```python
from build123d import *

# Parameters (mm, degrees)
ESQUISSE1_W                  = 53
ESQUISSE1_H                  = 38
BASE_DEPTH                   = 4
ESQUISSE2_W                  = 29
ESQUISSE2_H                  = 29
SCREEN_DEPTH                 = 4
ESQUISSE5_R                  = 2.25
INSERTS_M3_DEPTH             = 3
ESQUISSE6_W                  = 53
ESQUISSE6_H                  = 38
ESQUISSE6_W_2                = 50
ESQUISSE6_H_2                = 35
WALLS_DEPTH                  = 25
CHANFREIN_EXT_SIZE           = 1.2
CONG_1_R                     = 1.2
ESQUISSE7_R                  = 1.5
PASSAGE_VIS_HORIZONTAL_DEPTH = 62.603571325
ESQUISSE9_R                  = 1.5
PASSAGE_VIS_VERTICAL_DEPTH   = 53.642663306


with BuildPart() as part:
    # Esquisse1 → BASE (new body)
    with BuildSketch(Plane.XY):
        Rectangle(ESQUISSE1_W, ESQUISSE1_H)
    extrude(amount=BASE_DEPTH)

    # Esquisse2 → Screen (cut)
    with BuildSketch(Plane.XY.offset(4)):
        with Locations((-2.5, 0)):
            Rectangle(ESQUISSE2_W, ESQUISSE2_H)
    extrude(amount=-SCREEN_DEPTH, mode=Mode.SUBTRACT)

    # Esquisse5 → Inserts_M3 (cut)
    with BuildSketch(Plane(origin=(0, 0, 0), x_dir=(-1, 0, 0), z_dir=(0, 0, -1))):
        with Locations((-21, 13.5)):
            Circle(ESQUISSE5_R)
        with Locations(Location((-21, -13.5, 0), (0, 0, 180))):
            Circle(ESQUISSE5_R)
        with Locations((21, -13.5)):
            Circle(ESQUISSE5_R)
        with Locations(Location((21, 13.5, 0), (0, 0, 180))):
            Circle(ESQUISSE5_R)
    extrude(amount=-INSERTS_M3_DEPTH, mode=Mode.SUBTRACT)

    # Esquisse6 → Walls (add)
    with BuildSketch(Plane(origin=(0, 0, 0), x_dir=(-1, 0, 0), z_dir=(0, 0, -1))):
        Rectangle(ESQUISSE6_W, ESQUISSE6_H)
        Rectangle(ESQUISSE6_W_2, ESQUISSE6_H_2, mode=Mode.SUBTRACT)
    extrude(amount=WALLS_DEPTH)

    # Chanfrein_EXT
    chanfrein_ext_edges = [part.edges().sort_by_distance(p)[0] for p in [
        (26.5, 0, 4),
        (0, 19, 4),
        (-17, 0, 4),
        (-2.5, -14.5, 4),
        (12, 0, 4),
        (-2.5, 14.5, 4),
        (-26.5, 0, 4),
        (-26.5, 19, -10.5),
        (26.5, 19, -10.5),
        (26.5, -19, -10.5),
        (-26.5, -19, -10.5),
        (0, -19, 4),
    ]]
    chamfer(chanfrein_ext_edges, length=CHANFREIN_EXT_SIZE)

    # Congé1
    cong_1_edges = [part.edges().sort_by_distance(p)[0] for p in [
        (0, 17.5, 0),
        (25, 0, 0),
        (0, -17.5, 0),
        (-25, 0, 0),
        (25, 17.5, -12.5),
        (25, -17.5, -12.5),
        (-25, -17.5, -12.5),
        (-25, 17.5, -12.5),
    ]]
    fillet(cong_1_edges, radius=CONG_1_R)

    # Esquisse7 → Passage_Vis_Horizontal (cut, through all)
    with BuildSketch(Plane(origin=(26.5, 0, 0), x_dir=(0, 0, -1), z_dir=(1, 0, 0))):
        with Locations(Location((21, 0, 0), (0, 0, 90))):
            Circle(ESQUISSE7_R)
    extrude(amount=-PASSAGE_VIS_HORIZONTAL_DEPTH, mode=Mode.SUBTRACT)

    # Esquisse9 → Passage_Vis_Vertical (cut, through all)
    with BuildSketch(Plane(origin=(0, 19, 0), x_dir=(1, 0, 0), z_dir=(0, 1, 0))):
        with Locations(Location((-18.5, 21, 0), (0, 0, 180))):
            Circle(ESQUISSE9_R)
        with Locations(Location((18.5, 21, 0), (0, 0, 180))):
            Circle(ESQUISSE9_R)
    extrude(amount=-PASSAGE_VIS_VERTICAL_DEPTH, mode=Mode.SUBTRACT)


solid = part.part
```
Can you work these out from the model? Positions are in its coordinate system, mm. A direction names the side the tool comes from. Round coordinates to 2 decimals unless told otherwise and drop trailing zeros. Loops run counter-clockwise (first coordinate to the right, second up) from the corner with the lowest first, then second, coordinate; pieces in that order, holes last.
Item 1: If we mould it in two halves opening along Y, with no side actions, what happens to faces 1 (the flat face through (26.5, 0, -11)), 2 (the flat face through (0, 19, -11)), 3 (the cylindrical face through (-24.658, 0.228, -0.361))? For each: +Y half, -Y half, draft (parallel to the pull), parting line (faces both ways), or undercut.
Item 2: Suppose I cut it at A-A, the plane y = -13.5. Write out the boundary of the cut face in (x, z).
Item 3: Suppose I cut it at D-D, the plane z = -12. Write out the boundary of the cut face in (x, y), then the cut area to 3 significant figures.
Item 4: Please list where these lines run through material, in increasing order: L1, parallel to Y at x = -21, z = 2.2; L2, parallel to X at y = -7, z = 0.5; L3, parallel to X at y = -4, z = -12.
Item 5: Which directions (+Z, -Z, +X, -X, +Y, -Y) give clear straight access to the entire face, cutting with the end or side of a thin tool? Please do faces 4 (the cylindrical face through (-24.658, 17.139, -13.267)), 5 (the flat face through (-26.5, 0, -11)), 6 (the cylindrical face through (-17.39, -18.24, -19.99)), 7 (the flat face through (-3, -14.5, 1)), 8 (the flat face through (12.6, -0.2, 3.4)).
Item 6: Will these pins go through, and if not, where does the flat tip stop? pin 1 Ø5 at (x, y) = (20.5, -14.5) entering from -Z; pin 2 Ø16.5 at (x, y) = (-10.5, -8) entering from -Z.
Item 7: Suppose I cut it at C-C, the plane x = 9.5. Write out the boundary of the cut face in (y, z).
Item 8: Suppose I cut it at B-B, the plane y = 0. Write out the boundary of the cut face in (x, z), then the cut area to 3 significant figures.
Reported:
1. face 1: draft
1. face 2: +Y half
1. face 3: undercut
2. outline: (-26.5, -25) - (-25, -25) - (-25, -1.2) arc R1.2 cw to (-23.8, 0) - (-23.25, 0) - (-23.25, 3) - (-18.75, 3) - (-18.75, 0) - (-17, 0) - (-17, 2.8) - (-18.2, 4) - (-25.3, 4) - (-26.5, 2.8) - close; (12, 0) - (18.75, 0) - (18.75, 3) - (23.25, 3) - (23.25, 0) - (23.8, 0) arc R1.2 cw to (25, -1.2) - (25, -25) - (26.5, -25) - (26.5, 2.8) - (25.3, 4) - (13.2, 4) - (12, 2.8) - close
3. outline: (-26.5, -17.8) - (-25.3, -19) - (25.3, -19) - (26.5, -17.8) - (26.5, 17.8) - (25.3, 19) - (-25.3, 19) - (-26.5, 17.8) - close; hole (-25, -16.3) arc R1.2 ccw to (-23.8, -17.5) - (23.8, -17.5) arc R1.2 ccw to (25, -16.3) - (25, 16.3) arc R1.2 ccw to (23.8, 17.5) - (-23.8, 17.5) arc R1.2 ccw to (-25, 16.3) - close
3. area: 262 mm2
4. L1: y = -19 to -15.75, -11.25 to 11.25, 15.75 to 19
4. L2: x = -26.5 to -17, 12 to 26.5
4. L3: x = -26.5 to -25, 25 to 26.5
5. face 4: -Z
5. face 5: +Z, -Z, -X, +Y, -Y
5. face 6: +Y, -Y
5. face 7: +Z, -Z
5. face 8: +Z
6. pin 1: stops at z = -0.23
6. pin 2: stops at z = 0
7. outline: (-19, -25) - (-17.5, -25) - (-17.5, -1.2) arc R1.2 cw to (-16.3, 0) - (-14.5, 0) - (-14.5, 2.8) - (-15.7, 4) - (-17.8, 4) - (-19, 2.8) - close; (14.5, 0) - (16.3, 0) arc R1.2 cw to (17.5, -1.2) - (17.5, -25) - (19, -25) - (19, 2.8) - (17.8, 4) - (15.7, 4) - (14.5, 2.8) - close
8. outline: (-26.5, -25) - (-25, -25) - (-25, -22.5) - (-26.5, -22.5) - close; (-26.5, -19.5) - (-25, -19.5) - (-25, -1.2) arc R1.2 cw to (-23.8, 0) - (-17, 0) - (-17, 2.8) - (-18.2, 4) - (-25.3, 4) - (-26.5, 2.8) - close; (12, 0) - (23.8, 0) arc R1.2 cw to (25, -1.2) - (25, -19.5) - (26.5, -19.5) - (26.5, 2.8) - (25.3, 4) - (13.2, 4) - (12, 2.8) - close; (25, -25) - (26.5, -25) - (26.5, -22.5) - (25, -22.5) - close
8. area: 160 mm2
